Source: CAD feature listing. Evaluate the final solid. Frame: model axes, mm. A direction names the side the tool comes from. Give positions to 0.01 mm unless a question says otherwise; leave off trailing zeros. Write each loop counter-clockwise with the first axis right and the second up, starting at its lowest first coordinate (ties: lowest second). Pieces come first, ordered by that corner, then holes. Notation, with made-up numbers: (21, 58) -> (50, 58) arc R24 ccw to (50, 76) -> close; hole circle Ø1 at (26.25, -8.75). An arc over 180 degrees is marked (long way). Answer as a JSON object with one key per item and string values. Group by question number.
Item 1: Section query A-A on z = -2.75. Return the cut outline in (x, y).
Item 2: First-contact query: pin 1 Ø1 at (x, z) = (34.5, 1.5) entering from +Y; pin 2 Ø3 at (x, y) = (47.5, 4.5) entering from -Z; pin 3 Ø1.6 at (y, z) = (20.5, 1) entering from +X; pin 4 Ø4 at (x, y) = (0.89, 15.71) entering from -Z. Flat tips, straight axial feed; report the tip coordinate or a pass-through.
Item 3: Pull-direction query (Y, two-part tool) for faces 1 (the face through (50, 0, 1)), 2 (the face through (95.09, 14.97, 1.04)), 3 (the face through (99, 15, -9.5)); classes: pulls with the +Y half, pulls with the -Y half, needs draft (parallel to the pull), parting line crosses it, or undercut.
Item 4: Access query for faces 4 (the face through (6, 15, -8)), 5 (the face through (99.82, 15.17, -7.04)), 6 (the face through (98.65, 15, -4)), 7 (the face through (50.52, 27.09, 1.04)), 8 (the face through (102.3, 15, 1)). Directions: +Z, -Z, +X, -X, +Y, -Y. A direction counts if a zero-diameter tool reaches every point of the face in a straight line with its end or side. Return the directions, or none.
Item 5: Section query B-B on y = 9.5. Return the cut outline in (x, z), plus the area to 3 significant figures.
Item 6: Ray query, probe 1 along X at (y, z) = (16.5, -1.5); probe 2 along Y at (x, z) = (67.5, -0.75); probe 3 along X at (y, z) = (10, -8.5). Return the intervals inside material, ascending. Write a range as from..to.
Item 7: Section query C-C on x = 57. Return the cut outline in (y, z), plus the area to 3 significant figures.
from build123d import *

# Parameters (mm, degrees)
PAD_DEPTH       = 2
SKETCH001_W     = 86
SKETCH001_H     = 22
POCKET_DEPTH    = 5
SKETCH002_W     = 106.3
SKETCH002_H     = 34.3
SKETCH002_W_2   = 86
SKETCH002_H_2   = 22
PAD001_DEPTH    = 1
CHAMFER_SIZE    = 1.9
SKETCH003_W     = 5.65
SKETCH003_H     = 34.3
PAD002_DEPTH    = 6.5
SKETCH004_W     = 8
SKETCH004_H     = 34.3
PAD003_DEPTH    = 2
SKETCH005_R     = 1.6
POCKET001_DEPTH = 5


with BuildPart() as part:
    # Sketch → Pad (new body)
    with BuildSketch(Plane.XY):
        with BuildLine():
            Line((1, 0), (101.3, 0))
            ThreePointArc((101.3, 0), (102.007107, 0.292893), (102.3, 1))
            Line((102.3, 1), (102.3, 29.3))
            ThreePointArc((102.3, 29.3), (102.007107, 30.007107), (101.3, 30.3))
            Line((101.3, 30.3), (1, 30.3))
            ThreePointArc((1, 30.3), (0.292893, 30.007107), (0, 29.3))
            Line((0, 29.3), (0, 1))
            ThreePointArc((0, 1), (0.292893, 0.292893), (1, 0))
        make_face()
    extrude(amount=PAD_DEPTH)

    # Sketch001 (on Face10 of Pad) → Pocket (cut)
    with BuildSketch(Plane.XY.offset(2)):
        with Locations((51.15, 15.15)):
            Rectangle(SKETCH001_W, SKETCH001_H)
    extrude(amount=-POCKET_DEPTH, mode=Mode.SUBTRACT)

    # Sketch002 (on Face4 of Pocket) → Pad001 (join)
    with BuildSketch(Plane(origin=(0, 0, 0), x_dir=(1, 0, 0), z_dir=(0, 0, -1))):
        with Locations((51.15, -15.15)):
            Rectangle(SKETCH002_W, SKETCH002_H)
        with Locations((51.15, -15.15)):
            Rectangle(SKETCH002_W_2, SKETCH002_H_2, mode=Mode.SUBTRACT)
    extrude(amount=PAD001_DEPTH)

    # Chamfer
    chamfer_edges = [part.edges().sort_by_distance(p)[0] for p in [
        (51.15, 26.15, 2),
        (8.15, 15.15, 2),
        (51.15, 4.15, 2),
        (94.15, 15.15, 2),
    ]]
    chamfer(chamfer_edges, length=CHAMFER_SIZE)

    # Sketch003 (on Face27 of Chamfer) → Pad002 (join)
    with BuildSketch(Plane(origin=(0, 0, -1), x_dir=(1, 0, 0), z_dir=(0, 0, -1))):
        with Locations((101.475, -15.15)):
            Rectangle(SKETCH003_W, SKETCH003_H)
        with Locations((0.825, -15.15)):
            Rectangle(SKETCH003_W, SKETCH003_H)
    extrude(amount=PAD002_DEPTH)

    # Sketch004 (on Face36 of Pad002) → Pad003 (join)
    with BuildSketch(Plane(origin=(0, 0, -7.5), x_dir=(1, 0, 0), z_dir=(0, 0, -1))):
        with Locations((100.3, -15.15)):
            Rectangle(SKETCH004_W, SKETCH004_H)
        with Locations((2, -15.15)):
            Rectangle(SKETCH004_W, SKETCH004_H)
    extrude(amount=PAD003_DEPTH)

    # Sketch005 (on Face45 of Pad003) → Pocket001 (cut)
    with BuildSketch(Plane(origin=(0, 0, -9.5), x_dir=(1, 0, 0), z_dir=(0, 0, -1))):
        with Locations((0.89357, -15.708431)):
            Circle(SKETCH005_R)
        with Locations((101.41729, -15.243322)):
            Circle(SKETCH005_R)
    extrude(amount=-POCKET001_DEPTH, mode=Mode.SUBTRACT)


solid = part.part
Worked answers:
{
 "1": {"outline": "(-2, -2) -> (3.65, -2) -> (3.65, 32.3) -> (-2, 32.3) -> close; (98.65, -2) -> (104.3, -2) -> (104.3, 32.3) -> (98.65, 32.3) -> close"},
 "2": {"pin 1": "y = 30.3", "pin 2": "z = -1", "pin 3": "x = 102.3", "pin 4": "z = -9.5"},
 "3": {"face 1": "pulls with the -Y half", "face 2": "undercut", "face 3": "needs draft"},
 "4": {"face 4": "-Z, +Y, -Y", "face 5": "-Z", "face 6": "+Y, -Y", "face 7": "+Z", "face 8": "+Z, +X, +Y, -Y"},
 "5": {"outline": "(-2, -9.5) -> (6, -9.5) -> (6, -7.5) -> (3.65, -7.5) -> (3.65, -1) -> (8.15, -1) -> (8.15, 0.1) -> (6.25, 2) -> (0, 2) -> (0, 0) -> (-2, 0) -> close; (94.15, -1) -> (98.65, -1) -> (98.65, -7.5) -> (96.3, -7.5) -> (96.3, -9.5) -> (104.3, -9.5) -> (104.3, 0) -> (102.3, 0) -> (102.3, 2) -> (96.05, 2) -> (94.15, 0.1) -> close", "area": "155 mm^2"},
 "6": {"probe 1": "-2..3.65, 98.65..104.3", "probe 2": "-2..4.15, 26.15..32.3", "probe 3": "-2..6, 96.3..104.3"},
 "7": {"outline": "(-2, -1) -> (4.15, -1) -> (4.15, 0.1) -> (2.25, 2) -> (0, 2) -> (0, 0) -> (-2, 0) -> close; (26.15, -1) -> (32.3, -1) -> (32.3, 0) -> (30.3, 0) -> (30.3, 2) -> (28.05, 2) -> (26.15, 0.1) -> close", "area": "25.3 mm^2"}
}
